from build123d import *

# Parameters (mm, degrees)
F0_R     = 12.5312471482
F1_DEPTH = 2.5
F2_R     = 10.8098139949
F3_DEPTH = 75.98543


# Not quite as in the source:
# - a fillet or chamfer that OpenCascade refuses, or shapes differently, is made with other operations: its cross-section is extruded or revolved along the edge and cut away or added


with BuildPart() as f1:
    # F0 (on Front) → F1 (new body, symmetric)
    with BuildSketch(Plane.XZ):
        Circle(F0_R)
    extrude(amount=F1_DEPTH, both=True)

    # F2 (on face) → F3 (cut)
    with BuildSketch(Plane.XZ.offset(2.5)):
        Circle(F2_R)
    extrude(amount=-F3_DEPTH, mode=Mode.SUBTRACT)

    # F4: fillet of radius 2.5 on 1 edges, made by hand

    # F4_s1 → F4_t2 (revolve, cut)
    with BuildSketch(Plane.XY):
        with BuildLine():
            ThreePointArc((12.5312471482, -0.1243245876), (12.055650408, -1.5912231668), (10.8098139949, -2.5))
            Line((10.8098139949, -2.5), (12.5312471482, -2.5))
            Line((12.5312471482, -2.5), (12.5312471482, -0.1243245876))
        make_face()
    revolve(axis=Axis((0, -2.5, 0), (0, -1, 0)), mode=Mode.SUBTRACT)

    # F5: fillet of radius 2.5 on 1 edges, made by hand

    # F5_s1 → F5_t2 (revolve, cut)
    with BuildSketch(Plane.XY):
        with BuildLine():
            ThreePointArc((12.5312471482, 0.1243245876), (12.055650408, 1.5912231668), (10.8098139949, 2.5))
            Line((10.8098139949, 2.5), (12.5312471482, 2.5))
            Line((12.5312471482, 2.5), (12.5312471482, 0.1243245876))
        make_face()
    revolve(axis=Axis((0, 2.5, 0), (0, -1, 0)), mode=Mode.SUBTRACT)


solid = f1.part
Design review of the part built by this model. Coordinates are the model's own, in mm. Give positions to 0.01 mm unless a question says otherwise; leave off trailing zeros. Loops run counter-clockwise (first coordinate to the right, second up) from the corner with the lowest first, then second, coordinate; pieces in that order, holes last. Notation, with made-up numbers: M 21,-9 L 39,-9 A21 ccw 39,24 Z; hole C 54.25,63 d5. An arc over 180 degrees is marked long. Answer as a JSON object with one key per item and string values.
Item 1: For P1, Ø1, axis at y = -0.5, z = 8, coming from the -X side; P2, Ø4, axis at x = 8.5, z = -5, coming from the -Y side; P3, Ø1, axis at y = -0.5, z = 6.5, coming from the -X side, all flat-tipped, find the tip position at first contact; note any pin that passes through.
Output values:
{"P1": "stops at x = -10.01", "P2": "stops at y = -2.5", "P3": "stops at x = -10.98"}
Item 2: We need section C-C (y = -1.3). State the section outline as (x, z) points.
Output values:
{"outline": "C 0,0 d24.48; hole C 0,0 d21.62"}
Item 3: We need section A-A (x = 0). State the section outline as (y, z) points, and give its area (3 significant figures).
Output values:
{"outline": "M -2.5,-10.81 A2.5 ccw -0.12,-12.53 L 0.12,-12.53 A2.5 ccw 2.5,-10.81 Z; M -2.5,10.81 L 2.5,10.81 A2.5 ccw 0.12,12.53 L -0.12,12.53 A2.5 ccw Z", "area": "12.8 mm2"}
Item 4: Wall thickness on line 1 along Z through (x, y) = (0, 0.15); line 2 along X through (y, z) = (1.7, -4); line 3 along Z through (x, y) = (0, 0.85): over which ranges is each line inside the solid? List them lowest first.
Output values:
{"line 1": "z = -12.53 to -10.81, 10.81 to 12.53", "line 2": "x = -11.28 to -10.04, 10.04 to 11.28", "line 3": "z = -12.42 to -10.81, 10.81 to 12.42"}
Item 5: We need section B-B (z = 0). State the section outline as (x, y) points, and give its area (3 significant figures).
Output values:
{"outline": "M -12.53,-0.12 A2.5 ccw -10.81,-2.5 L -10.81,2.5 A2.5 ccw -12.53,0.12 Z; M 10.81,-2.5 A2.5 ccw 12.53,-0.12 L 12.53,0.12 A2.5 ccw 10.81,2.5 Z", "area": "12.8 mm2"}
Item 6: We need section D-D (y = 1.9). State the section outline as (x, z) points, and give its area (3 significant figures).
Output values:
{"outline": "C 0,0 d23.58; hole C 0,0 d21.62", "area": "69.7 mm2"}
